from build123d import *

# Parameters (mm, degrees)
SKETCH1_R              = 16.1
SKETCH1_R_2            = 4
BOSS_EXTRUDE1_DEPTH    = 2
SKETCH2_R              = 20.1
SKETCH2_R_2            = 16.1
BOSS_EXTRUDE2_DEPTH    = 10
CUT_SWEEP2_PITCH       = 12
CUT_SWEEP2_HEIGHT      = 3
CUT_SWEEP2_RADIUS      = 16.1
CUT_SWEEP2_START_ANGLE = -90
SKETCH35_W             = 3.2
SKETCH35_H             = 2
CIRPATTERN3_COUNT      = 4
CUT_EXTRUDE1_DEPTH     = 2
CIRPATTERN4_COUNT      = 4
CUT_EXTRUDE4_DEPTH     = 3
CIRPATTERN5_COUNT      = 4


with BuildPart() as part:
    # Sketch1 → Boss-Extrude1 (new body)
    with BuildSketch(Plane(origin=(0, 0, 0), x_dir=(1, 0, 0), z_dir=(0, 1, 0))):
        Circle(SKETCH1_R)
        Circle(SKETCH1_R_2, mode=Mode.SUBTRACT)
        with BuildLine():
            ThreePointArc((12, 0), (0, 12), (-12, 0))
            ThreePointArc((-12, 0), (-10, -2), (-8, 0))
            ThreePointArc((-8, 0), (0, 8), (8, 0))
            ThreePointArc((8, 0), (10, -2), (12, 0))
        make_face(mode=Mode.SUBTRACT)
    extrude(amount=BOSS_EXTRUDE1_DEPTH)

    # Sketch2 → Boss-Extrude2 (add)
    with BuildSketch(Plane(origin=(0, 0, 0), x_dir=(1, 0, 0), z_dir=(0, 1, 0))):
        Circle(SKETCH2_R)
        Circle(SKETCH2_R_2, mode=Mode.SUBTRACT)
    extrude(amount=BOSS_EXTRUDE2_DEPTH)

    # Cut-Sweep2: sweep along a helix
    with BuildLine() as cut_sweep2_path:
        add(Helix(CUT_SWEEP2_PITCH, CUT_SWEEP2_HEIGHT, CUT_SWEEP2_RADIUS, center=(0, 8, 0), direction=(0, -1, 0), mode=Mode.PRIVATE).rotate(Axis((0, 8, 0), (0, -1, 0)), CUT_SWEEP2_START_ANGLE))
    # Sketch35 → Cut-Sweep2 (sweep, cut)
    with BuildSketch(Plane.XY):
        with Locations((-16.1, 8)):
            Rectangle(SKETCH35_W, SKETCH35_H)
    cut_sweep2 = sweep(path=cut_sweep2_path.line, is_frenet=True, mode=Mode.SUBTRACT)

    # CirPattern3: Cut-Sweep2 ×4 about axis
    cirpattern3_axis = Axis((0, 2, 0), (0, -1, 0))
    for i in range(1, CIRPATTERN3_COUNT):
        add(cut_sweep2.rotate(cirpattern3_axis, i * 360 / CIRPATTERN3_COUNT), mode=Mode.SUBTRACT)

    # Sketch36 → Cut-Extrude1 (cut)
    with BuildSketch(Plane(origin=(0, 10, 0), x_dir=(1, 0, 0), z_dir=(0, 1, 0))):
        with BuildLine():
            Line((-17.7, 0), (-16.1, 0))
            ThreePointArc((-16.1, 0), (-15.975293425, 2), (-15.60310559, 3.969017))
            Line((-15.60310559, 3.969017), (-17.182789415, 4.247557879))
            ThreePointArc((-17.182789415, 4.247557879), (-17.570221579, 2.139465747), (-17.7, 0))
        make_face()
    cut_extrude1 = extrude(amount=-CUT_EXTRUDE1_DEPTH, mode=Mode.SUBTRACT)

    # CirPattern4: Cut-Extrude1 ×4 about axis
    cirpattern4_axis = Axis((0, 0, 0), (0, 1, 0))
    for i in range(1, CIRPATTERN4_COUNT):
        add(cut_extrude1.rotate(cirpattern4_axis, i * 360 / CIRPATTERN4_COUNT), mode=Mode.SUBTRACT)

    # Sketch37 → Cut-Extrude4 (cut)
    with BuildSketch(Plane(origin=(0, 2, 0), x_dir=(1, 0, 0), z_dir=(0, 1, 0))):
        with BuildLine():
            Line((-15.129051195, 5.506524308), (-16.632559388, 6.053756537))
            ThreePointArc((-16.632559388, 6.053756537), (-17.674804761, 0.944074504), (-17.182789415, -4.247557879))
            Line((-17.182789415, -4.247557879), (-15.60310559, -3.969017))
            ThreePointArc((-15.60310559, -3.969017), (-16.079889176, 0.804465085), (-15.129051195, 5.506524308))
        make_face()
    cut_extrude4 = extrude(amount=CUT_EXTRUDE4_DEPTH, mode=Mode.SUBTRACT)

    # CirPattern5: Cut-Extrude4 ×4 about axis
    cirpattern5_axis = Axis((0, 0, 0), (0, 1, 0))
    for i in range(1, CIRPATTERN5_COUNT):
        add(cut_extrude4.rotate(cirpattern5_axis, i * 360 / CIRPATTERN5_COUNT), mode=Mode.SUBTRACT)


solid = part.part
Verification items for the finished model (mm, model axes). A direction names the side the tool comes from. Give positions to 0.01 mm unless a question says otherwise; leave off trailing zeros. Order: outer loops, then holes, each group sorted by start corner. A loop starts at its lowest first (then second) coordinate and runs counter-clockwise, first axis right, second up. Notation, with made-up numbers: (78, 67) -> (102, 67) arc R23 ccw to (102, 85) -> close; hole circle Ø3 at (-7, 69). An arc over 180 degrees is marked (long way). Answer as CSV lines item,"result".
Q1. Sectioned sample at B-B on x = 3. Count the separate pieces of the cut face and the enclosed holes in it, plus the area to 3 significant figures.
Solutions:
separate pieces,"3"
enclosed holes,"0"
area,"108 mm²"
Q2. Depth check by flat-ended pin: pin 1 (1.3 mm diameter, centred on x = -17, y = 8, fed in from -Z); pin 2 (1.5 mm diameter, centred on y = 9, z = -12.5, fed in from -X); pin 3 (1.5 mm diameter, centred on x = -12.5, z = -4, fed in from +Y). Enter the tip coordinate at first touch or a pass-through.
Solutions:
pin 1,"stops at z = -11.69"
pin 2,"stops at x = -16.31"
pin 3,"stops at y = 2"
Q3. Release check for a two-part mould opening along X. For faces 1 (the cylindrical face through (17.67, 3.48, 1.02)), 2 (the cylindrical face through (19.17, 4.93, -6.04)) record: +X half, -X half, draft (parallel to the pull), parting line (faces both ways), or undercut.
Solutions:
face 1,"undercut"
face 2,"parting line"
Q4. Access from +Z, -Z, +X, -X, +Y, -Y to the whole of each face (thin tool, end or side, straight path). Record for faces 3 (the flat face through (3, 5, -16)), 4 (the flat face through (-17, 9, 0)), 5 (the cylindrical face through (10, 1, 2)).
Solutions:
face 3,"none"
face 4,"+Y"
face 5,"+Y, -Y"
Q5. Scan lines: probe 1 along Z at (x, y) = (0, 0.6); probe 2 along X at (y, z) = (2.75, 0); probe 3 along Y at (x, z) = (-9.5, -11). Record each from-to range of solid material in increasing order.
Solutions:
probe 1,"z = -20.1 to -12, -8 to -4, 4 to 20.1"
probe 2,"x = -20.1 to -17.7, 17.7 to 20.1"
probe 3,"y = 0 to 2"
Q6. Sectioned sample at A-A on y = 9.5. Record the cut outline in (x, z), plus the area to 3 significant figures.
Solutions:
outline,"circle Ø40.2 at (0, 0); hole (-17.7, 0) arc R17.7 ccw to (-17.18, -4.25) -> (-15.6, -3.97) arc R16.1 ccw to (0, -16.1) -> (0, -17.7) arc R17.7 ccw to (4.25, -17.18) -> (3.97, -15.6) arc R16.1 ccw to (16.1, 0) -> (17.7, 0) arc R17.7 ccw to (17.18, 4.25) -> (15.6, 3.97) arc R16.1 ccw to (0, 16.1) -> (0, 17.7) arc R17.7 ccw to (-4.25, 17.18) -> (-3.97, 15.6) arc R16.1 ccw to (-16.1, 0) -> close"
area,"428 mm²"
